The model under review builds one solid part; all positions refer to its coordinate system, in mm. Face numbers are marked on the shaded views. Round coordinates to 2 decimals unless told otherwise and drop trailing zeros. Order: outer loops, then holes, each group sorted by start corner. A loop starts at its lowest first (then second) coordinate and runs counter-clockwise, first axis right, second up.
1) Consider section A-A (y = 0). Give the boundary of the cut face in (x, z) (1 decimal), then the cut area to 3 significant figures.
2) Consider section C-C (z = 9). Give the boundary of the cut face in (x, y) (3 decimals).
3) Clearance check with flat-ended pins moving along their axes: P1, Ø3, axis at y = 21.5, z = 26, coming from the -X side; P2, Ø8, axis at x = -26, y = -11, coming from the -Z side; P3, Ø5, axis at x = 11, y = 12, coming from the -Z side; P4, Ø1, axis at y = -14, z = 23.5, coming from the +X side. State where each tip first meets the part, or that it passes through.
4) Mouldability with a two-part tool opening along Y and no side actions: class the marked faces 1 and 2 as pulls with the +Y half, pulls with the -Y half, needs draft (parallel to the pull), parting line crosses it, or undercut.
5) To check wall thickness, follow L1, parallel to Y at x = 0, z = 34.75; L2, parallel to Y at x = 13.5, z = 29; L3, parallel to X at y = 18, z = 29.5. State the ranges of each line that lie inside material, in increasing order.
6) Consider section B-B (x = 0). Give the number of separate pieces and of enclosed holes in the cut face, then the cut area to 3 significant figures.
7) Consider section D-D (z = 30). Give the boundary of the cut face in (x, y), then the cut area to 3 significant figures.
from build123d import *

# Parameters (mm, degrees)
F0_W     = 1.5875
F0_H     = 12.7
F2_R     = 2.38125
F3_DEPTH = 32.9692
F4_R     = 43.342469
F5_DEPTH = 1.27


with BuildPart() as f1:
    # F0 (on Front) → F1 (revolve)
    with BuildSketch(Plane.XZ):
        Polygon((30.6705, 25.4), (20.955, 25.4), (20.955, 0), (33.02, 25.4), (32.258, 25.4), align=None)
        with Locations((31.46425, 31.75)):
            Rectangle(F0_W, F0_H)
    revolve(axis=Axis((0, 0, 24.195854), (0, 0, 1)))

    # F2 (on face) → F3 (cut)
    with BuildSketch(Plane.XY.offset(25.4)):
        with Locations((0, -28.159229)):
            Circle(F2_R)
    extrude(amount=-F3_DEPTH, mode=Mode.SUBTRACT)

    # F4 (on Top) → F5 (cut)
    with BuildSketch(Plane.XY):
        Circle(F4_R)
    extrude(amount=F5_DEPTH, mode=Mode.SUBTRACT)


solid = f1.part
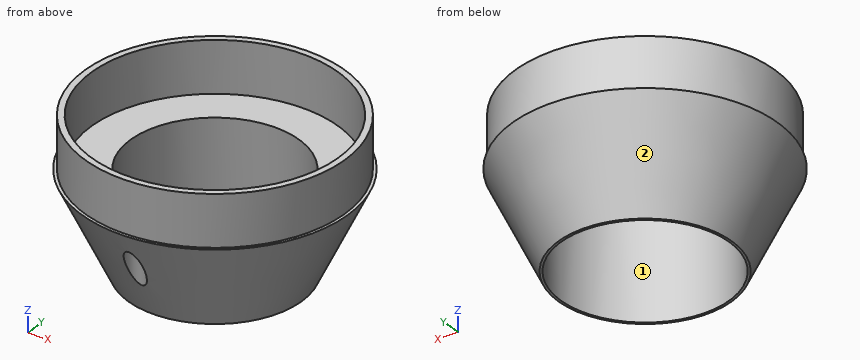
Answer below:
1. outline: (-33, 25.4) - (-21.6, 1.3) - (-21, 1.3) - (-21, 25.4) - (-30.7, 25.4) - (-30.7, 38.1) - (-32.3, 38.1) - (-32.3, 25.4) - close; (21, 1.3) - (21.6, 1.3) - (33, 25.4) - (32.3, 25.4) - (32.3, 38.1) - (30.7, 38.1) - (30.7, 25.4) - (21, 25.4) - close
1. area: 346 mm2
2. outline: circle Ø50.46 at (0, 0); hole circle Ø41.91 at (0, 0)
3. P1: stops at x = -26.18
3. P2: stops at z = 6.9
3. P3: passes through
3. P4: stops at x = 29.26
4. face 1: undercut
4. face 2: parting line crosses it
5. L1: y = -32.26 to -30.67, 30.67 to 32.26
5. L2: y = -29.3 to -27.54, 27.54 to 29.3
5. L3: x = -26.77 to -24.83, 24.83 to 26.77
6. separate pieces: 3
6. enclosed holes: 0
6. area: 297 mm2
7. outline: circle Ø64.52 at (0, 0); hole circle Ø61.34 at (0, 0)
7. area: 314 mm2
